```python
from build123d import *
from build123d.topology import SkipClean

# Parameters (mm, degrees)
SKETCH1_R                            = 15
SKETCH1_R_2                          = 8
BOSS_EXTRUDE1_DEPTH                  = 30
SKETCH3_R                            = 15
SKETCH3_R_2                          = 8
BOSS_EXTRUDE3_DEPTH                  = 30
BOSS_EXTRUDE4_REACH                  = 75.485
BOSS_EXTRUDE4_END_RADIUS             = 15
SKETCH4_R                            = 10
BOSS_EXTRUDE4_DIRECTION_2_REACH      = 75.485
BOSS_EXTRUDE4_DIRECTION_2_END_RADIUS = 15


with BuildPart() as part:
    # Sketch1 → Boss-Extrude1 (new, symmetric)
    with BuildSketch(Plane(origin=(0, 0, 0), x_dir=(1, 0, 0), z_dir=(0, 1, 0))):
        with Locations(Location((0, 0, 0), (0, 0, 270))):
            Circle(SKETCH1_R)
        with Locations(Location((0, 0, 0), (0, 0, 270))):
            Circle(SKETCH1_R_2, mode=Mode.SUBTRACT)
    extrude(amount=BOSS_EXTRUDE1_DEPTH, both=True)



with BuildPart() as body_2:
    # Sketch3 → Boss-Extrude3 (new, symmetric)
    with BuildSketch(Plane.XY):
        with Locations((60, 0)):
            Circle(SKETCH3_R)
        with Locations((60, 0)):
            Circle(SKETCH3_R_2, mode=Mode.SUBTRACT)
    extrude(amount=BOSS_EXTRUDE3_DEPTH, both=True)


with BuildPart() as part_1:
    add(part.part)

    add(body_2.part)  # Boss-Extrude4 merges body 2
    # Boss-Extrude4: up to this cylinder (the profile starts outside it)
    boss_extrude4_end = Plane(origin=(60, 0, 0), z_dir=(0, 0, -1)) * Cylinder(BOSS_EXTRUDE4_END_RADIUS, 181.97, mode=Mode.PRIVATE)
    # Sketch4 → Boss-Extrude4 (add, up to the surface)
    with BuildSketch(Plane(origin=(15, 0, 0), x_dir=(0, 0, -1), z_dir=(1, 0, 0)), mode=Mode.PRIVATE) as boss_extrude4_sk1:
        with Locations(Location((0, 0, 0), (0, 0, 180))):
            Circle(SKETCH4_R)
    boss_extrude4_tool1 = extrude(boss_extrude4_sk1.sketch, amount=BOSS_EXTRUDE4_REACH, mode=Mode.PRIVATE) - boss_extrude4_end
    add(boss_extrude4_tool1.solids().sort_by_distance((15, 0, 0))[0])

    # Boss-Extrude4 direction 2: up to this cylinder (the profile starts outside it)
    with SkipClean():  # the faces are left unmerged after this step: merging them gives an invalid solid
        boss_extrude4_direction_2_end = Plane(origin=(0, 0, 0), z_dir=(0, -1, 0)) * Cylinder(BOSS_EXTRUDE4_DIRECTION_2_END_RADIUS, 181.97, mode=Mode.PRIVATE)
        # Sketch4 → Boss-Extrude4 direction 2 (add, up to the surface)
        with BuildSketch(Plane(origin=(15, 0, 0), x_dir=(0, 0, -1), z_dir=(1, 0, 0)), mode=Mode.PRIVATE) as boss_extrude4_direction_2_sk1:
            with Locations(Location((0, 0, 0), (0, 0, 180))):
                Circle(SKETCH4_R)
        boss_extrude4_direction_2_tool1 = extrude(boss_extrude4_direction_2_sk1.sketch, amount=-BOSS_EXTRUDE4_DIRECTION_2_REACH, mode=Mode.PRIVATE) - boss_extrude4_direction_2_end
        add(boss_extrude4_direction_2_tool1.solids().sort_by_distance((15, 0, 0))[0])
        add(boss_extrude4_direction_2_tool1.solids().sort_by_distance((15, 0, 0))[1])


solid = part_1.part
```
Can you work these out from the model? Positions are in its coordinate system, mm. Round coordinates to 2 decimals unless told otherwise and drop trailing zeros. Loops run counter-clockwise (first coordinate to the right, second up) from the corner with the lowest first, then second, coordinate; pieces in that order, holes last.
Item 1: If we mould it in two halves opening along X, with no side actions, what happens to faces 1 (the cylindrical face through (-14.643, 0.42, -3.252)), 2 (the flat face through (66, -6, 30))? For each: +X half, -X half, draft (parallel to the pull), parting line (faces both ways), or undercut.
Item 2: Suppose I cut it at D-D, the plane z = -2. Write out the boundary of the cut face in (x, y).
Item 3: Suppose I cut it at A-A, the plane x = 0. Write out the boundary of the cut face in (y, z).
Item 4: Suppose I cut it at C-C, the plane z = -14. Write out the boundary of the cut face in (x, y).
Item 5: Will these pins go through, and if not, where does the flat tip stop? pin 1 Ø10 at (x, y) = (18, 21.5) entering from -Z; pin 2 Ø1.5 at (x, y) = (18.5, -6.5) entering from +Z; pin 3 Ø13 at (x, y) = (60, 0) entering from +Z; pin 4 Ø3 at (x, z) = (33, -5) entering from +Y.
Item 6: Suppose I cut it at B-B, the plane y = -14. Write out the boundary of the cut face in (x, z).
Item 7: Please list where these lines run through material, in increasing order: L1, parallel to X at y = -13, z = -3; L2, parallel to X at y = -6.5, z = 0; L3, parallel to X at y = -3, z = -27.
Reported:
1. face 1: undercut
1. face 2: draft
2. outline: (-14.87, -30) - (-7.75, -30) - (-7.75, 30) - (-14.87, 30) - close; (7.75, -30) - (14.87, -30) - (14.87, -9.8) - (48.64, -9.8) arc R15 ccw (long way) to (48.64, 9.8) - (14.87, 9.8) - (14.87, 30) - (7.75, 30) - close; hole circle Ø16 at (60, 0)
3. outline: (-30, -15) - (30, -15) - (30, -8) - (-30, -8) - close; (-30, 8) - (30, 8) - (30, 15) - (-30, 15) - close
4. outline: (-5.39, -30) - (5.39, -30) - (5.39, 30) - (-5.39, 30) - close; circle Ø30 at (60, 0); hole circle Ø16 at (60, 0)
5. pin 1: stops at z = -7.48
5. pin 2: stops at z = 8.18
5. pin 3: passes through
5. pin 4: stops at y = 9.37
6. outline: circle Ø30 at (0, 0); (54.61, -30) - (65.39, -30) - (65.39, 30) - (54.61, 30) - close; hole circle Ø16 at (0, 0)
7. L1: x = -14.7 to -7.42, 7.42 to 14.7, 52.52 to 67.48
7. L2: x = -15 to -8, 8 to 55.34, 64.66 to 73.52
7. L3: x = 45.3 to 52.58, 67.42 to 74.7
